Here's how the part is built. I have some questions about the finished solid (model axes, mm). Face numbers are marked on the shaded views. A direction names the side the tool comes from. Coordinates: 2 decimals unless noted, no trailing zeros. Loops run counter-clockwise (first coordinate to the right, second up) from the corner with the lowest first, then second, coordinate; pieces in that order, holes last. Notation, with made-up numbers: (45.25, 30.5) -> (85.25, 30.5) arc R35 cw to (85.25, 67.5) -> close; hole circle Ø6 at (-29.75, 31). An arc over 180 degrees is marked (long way). Answer as a JSON object with one key per item and string values. Group by question number.
Q1. Thinking about a two-plate mould opening in X: for the marked faces 1, 2 and 3, which applies, released by +X, released by -X, zero draft, split by the parting line, or undercut?
Q2. I want a section at B-B on y = 6.5. Write out the boundary of the cut face in (x, z), then the cut area to 3 significant figures.
Q3. I'm going to push a flat-ended pin straight in: pin 1 (1.4 mm diameter, centred on x = -33.5, z = 4, fed in from -Y). Where does the tip first touch, or does it pass through?
Q4. I want a section at A-A on x = -28.5. Write out the boundary of the cut face in (y, z).
Q5. I need wall thicknesses on line 1 (X direction, y = 4, z = 3.05); line 2 (X direction, y = -2.5, z = 0.7); line 3 (Y direction, x = -31.5, z = 4.55). Which ranges of each line are inside material? Lowest first, please.
Q6. On a 3-axis mill with a long thin cutter (end or side, diameter ignored), from which of +Z, -Z, +X, -X, +Y, -Y can I reach the whole of each face in a straight line? I mean the marked faces 4, 5 and 6. Say none if no direction works.
Q7. I want a section at C-C on z = 0.75. Write out the boundary of the cut face in (x, y).
```python
from build123d import *

# Parameters (mm, degrees)
SKETCH2_R           = 0.8636
BOSS_EXTRUDE1_DEPTH = 5.842
SKETCH4_W           = 22.86
SKETCH4_H           = 3.81
BOSS_EXTRUDE2_DEPTH = 5.842
CUT_EXTRUDE1_DEPTH  = 45.657083246


with BuildPart() as part:
    # Sketch2 → Boss-Extrude1 (new body)
    with BuildSketch(Plane.XY):
        Polygon((-42.70375, -5.842), (-35.71875, -5.842), (-35.71875, 0), (-26.82875, 0), (-26.82875, -5.842), (-19.84375, -5.842), (-19.84375, 7.874), (-42.70375, 7.874), align=None)
        with Locations((-39.78275, 4.953)):
            Circle(SKETCH2_R, mode=Mode.SUBTRACT)
        with Locations(Location((-22.76475, 4.953, 0), (0, 0, 180))):
            Circle(SKETCH2_R, mode=Mode.SUBTRACT)
    extrude(amount=BOSS_EXTRUDE1_DEPTH)

    # Sketch4 → Boss-Extrude2 (add)
    with BuildSketch(Plane.XY.offset(5.842)):
        with Locations((-31.27375, 9.779)):
            Rectangle(SKETCH4_W, SKETCH4_H)
    extrude(amount=-BOSS_EXTRUDE2_DEPTH)

    # Sketch3 → Cut-Extrude1 (cut, through all)
    with BuildSketch(Plane.XY.offset(5.842)):
        Polygon((-32.73425, 0), (-32.73425, 4.5212), (-34.44875, 4.5212), (-34.44875, 6.858), (-32.73425, 6.858), (-32.73425, 8.128), (-29.81325, 8.128), (-29.81325, 6.858), (-28.09875, 6.858), (-28.09875, 4.5212), (-29.81325, 4.5212), (-29.81325, 0), align=None)
    extrude(amount=-CUT_EXTRUDE1_DEPTH, mode=Mode.SUBTRACT)


solid = part.part
```
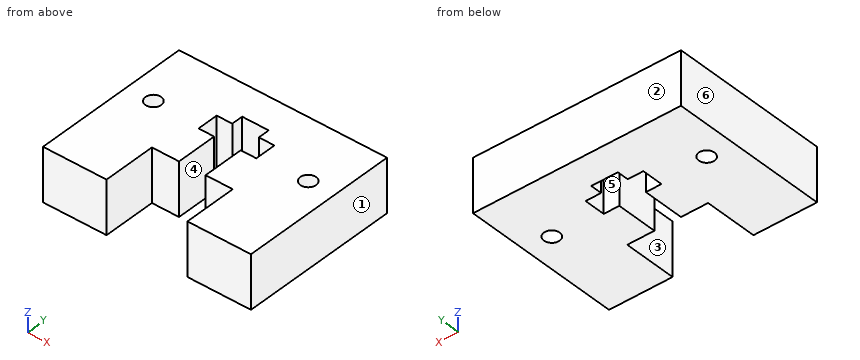
Result set:
{
 "1": {"face 1": "released by +X", "face 2": "zero draft", "face 3": "undercut"},
 "2": {"outline": "(-42.7, 0) -> (-34.45, 0) -> (-34.45, 5.84) -> (-42.7, 5.84) -> close; (-28.1, 0) -> (-19.84, 0) -> (-19.84, 5.84) -> (-28.1, 5.84) -> close", "area": "96.5 mm²"},
 "3": {"pin 1": "stops at y = 0"},
 "4": {"outline": "(0, 0) -> (4.52, 0) -> (4.52, 5.84) -> (0, 5.84) -> close; (6.86, 0) -> (11.68, 0) -> (11.68, 5.84) -> (6.86, 5.84) -> close"},
 "5": {"line 1": "x = -42.7 to -32.73, -29.81 to -19.84", "line 2": "x = -42.7 to -35.72, -26.83 to -19.84", "line 3": "y = 8.13 to 11.68"},
 "6": {"face 4": "+Z, -Z, -Y", "face 5": "+Z, -Z", "face 6": "+Z, -Z, -X, +Y, -Y"},
 "7": {"outline": "(-42.7, -5.84) -> (-35.72, -5.84) -> (-35.72, 0) -> (-32.73, 0) -> (-32.73, 4.52) -> (-34.45, 4.52) -> (-34.45, 6.86) -> (-32.73, 6.86) -> (-32.73, 8.13) -> (-29.81, 8.13) -> (-29.81, 6.86) -> (-28.1, 6.86) -> (-28.1, 4.52) -> (-29.81, 4.52) -> (-29.81, 0) -> (-26.83, 0) -> (-26.83, -5.84) -> (-19.84, -5.84) -> (-19.84, 11.68) -> (-42.7, 11.68) -> close; hole circle Ø1.73 at (-39.78, 4.95); hole circle Ø1.73 at (-22.76, 4.95)"}
}
